Check sheet for the drawn part. Datum: minimum x, y, z corner. Units: mm. A direction names the side the tool comes from. Round coordinates to 2 decimals unless told otherwise and drop trailing zeros. Order: outer loops, then holes, each group sorted by start corner. A loop starts at its lowest first (then second) coordinate and runs counter-clockwise, first axis right, second up. Notation, with made-up numbers: (65.25, -8) -> (119.25, -8) arc R22 ccw to (119.25, 1) -> close; hole circle Ø10 at (0, 0). An arc over 180 degrees is marked (long way). Answer in a Markdown table with one row per item.
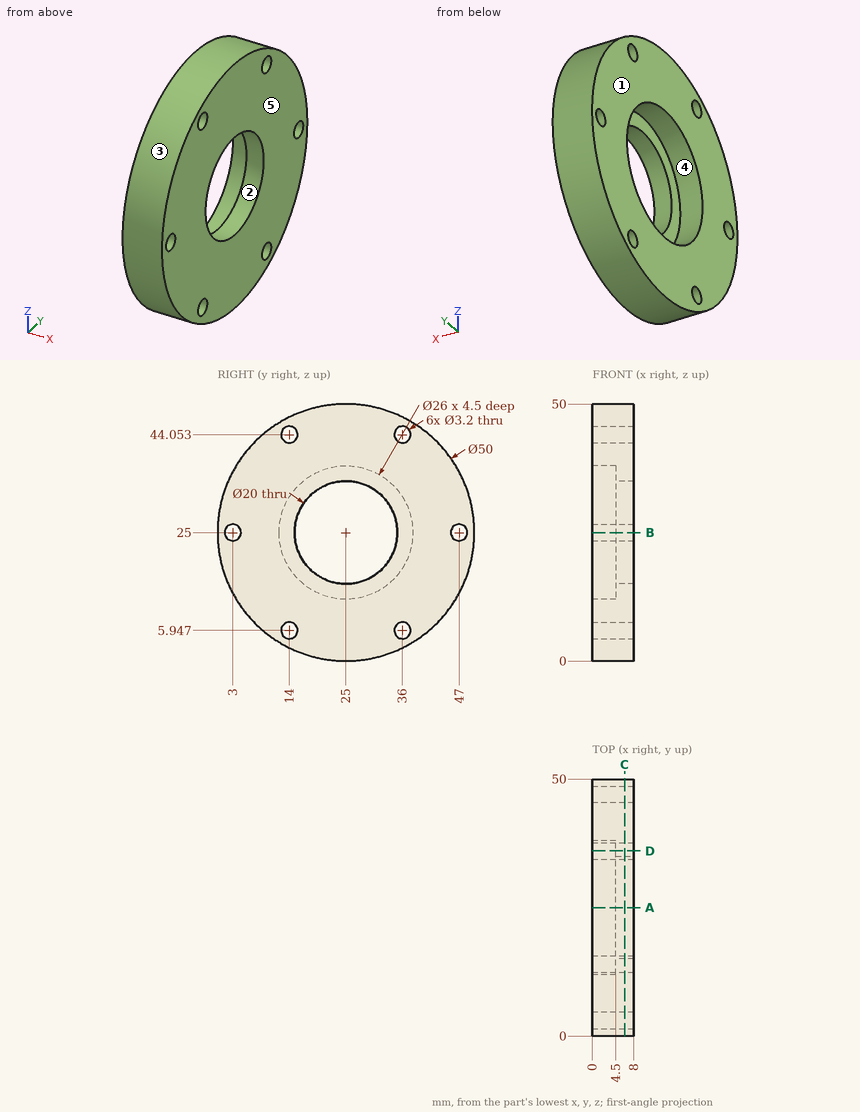
(1) Section check C-C on x = 6.25. Record the boundary of the cut face in (y, z).
Solutions:
| item | result |
|---|---|
| outline | circle Ø50 at (25, 25); hole circle Ø3.2 at (3, 25); hole circle Ø3.2 at (14, 5.95); hole circle Ø3.2 at (14, 44.05); hole circle Ø20 at (25, 25); hole circle Ø3.2 at (36, 5.95); hole circle Ø3.2 at (36, 44.05); hole circle Ø3.2 at (47, 25) |
(2) Section check B-B on z = 25. Record the boundary of the cut face in (x, y), plus the area to 3 significant figures.
Solutions:
| item | result |
|---|---|
| outline | (0, 0) -> (8, 0) -> (8, 1.4) -> (0, 1.4) -> close; (0, 4.6) -> (8, 4.6) -> (8, 15) -> (4.5, 15) -> (4.5, 12) -> (0, 12) -> close; (0, 38) -> (4.5, 38) -> (4.5, 35) -> (8, 35) -> (8, 45.4) -> (0, 45.4) -> close; (0, 48.6) -> (8, 48.6) -> (8, 50) -> (0, 50) -> close |
| area | 162 mm^2 |
(3) Section check D-D on y = 36. Record the boundary of the cut face in (x, z).
Solutions:
| item | result |
|---|---|
| outline | (0, 2.55) -> (8, 2.55) -> (8, 4.35) -> (0, 4.35) -> close; (0, 7.55) -> (8, 7.55) -> (8, 42.45) -> (0, 42.45) -> (0, 31.93) -> (4.5, 31.93) -> (4.5, 18.07) -> (0, 18.07) -> close; (0, 45.65) -> (8, 45.65) -> (8, 47.45) -> (0, 47.45) -> close |
(4) Draft check along Z on the marked faces 1, 2 and 3. Enter one of: pulls with the +Z half, pulls with the -Z half, needs draft (parallel to the pull), parting line crosses it, or undercut.
Solutions:
| item | result |
|---|---|
| face 1 | needs draft |
| face 2 | undercut |
| face 3 | parting line crosses it |
(5) Section check A-A on y = 25. Record the boundary of the cut face in (x, z).
Solutions:
| item | result |
|---|---|
| outline | (0, 0) -> (8, 0) -> (8, 15) -> (4.5, 15) -> (4.5, 12) -> (0, 12) -> close; (0, 38) -> (4.5, 38) -> (4.5, 35) -> (8, 35) -> (8, 50) -> (0, 50) -> close |
(6) Depth check by flat-ended pin: pin 1 Ø4 at (y, z) = (36, 44.05) entering from -X; pin 2 Ø3 at (x, z) = (2.5, 33.5) entering from +Y; pin 3 Ø8 at (y, z) = (30.5, 22) entering from -X; pin 4 Ø3 at (x, z) = (5, 31.5) entering from +Y (1 decimal). Enter the tip coordinate at first touch or a pass-through.
Solutions:
| item | result |
|---|---|
| pin 1 | x = 0 |
| pin 2 | y = 49 |
| pin 3 | x = 4.5 |
| pin 4 | y = 49.5 |
(7) Tool access check on the marked faces 4 and 5. Record the directions out of +Z, -Z, +X, -X, +Y, -Y that give a thin tool (end or side, any length) a straight path to the whole face; none if there is none.
Solutions:
| item | result |
|---|---|
| face 4 | -X |
| face 5 | +Z, -Z, +X, +Y, -Y |
(8) Scan lines: probe 1 along Z at (x, y) = (5, 14); probe 2 along Z at (x, y) = (1.8, 25); probe 3 along X at (y, z) = (32, 15.5). Record each from-to range of solid material in increasing order. Write a range as from..to.
Solutions:
| item | result |
|---|---|
| probe 1 | 2.55..4.35, 7.55..42.45, 45.65..47.45 |
| probe 2 | 0..12, 38..50 |
| probe 3 | 4.5..8 |
